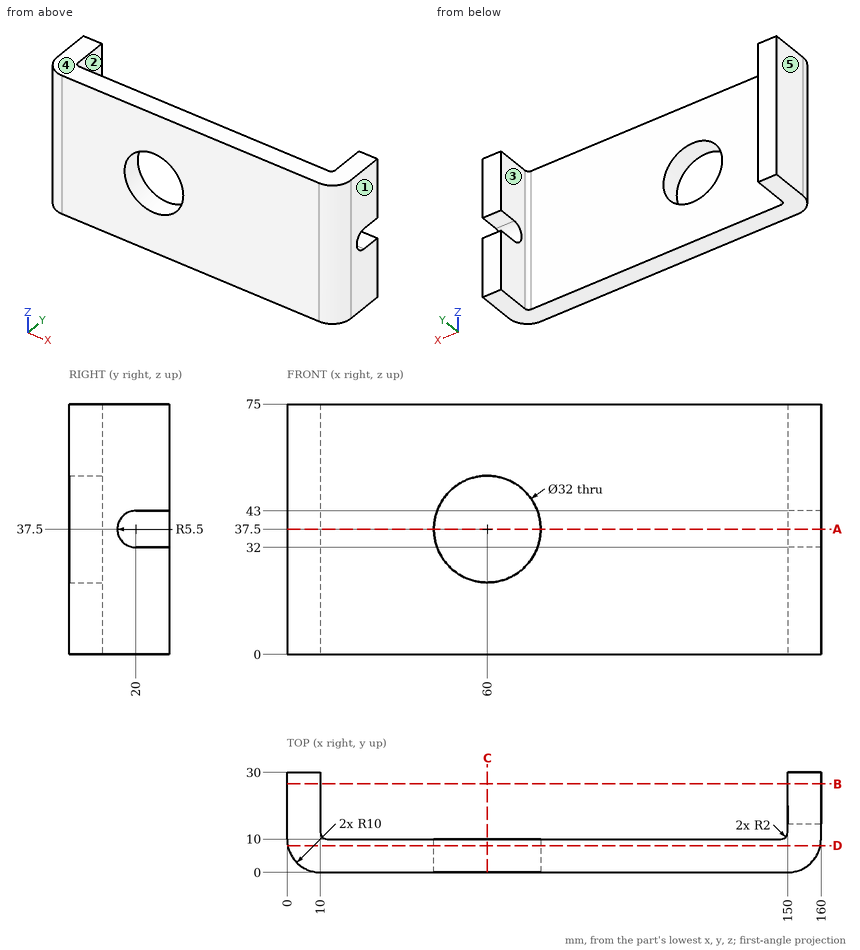
Check sheet for the drawn part. Datum: minimum x, y, z corner. Units: mm. A direction names the side the tool comes from. Give positions to 0.01 mm unless a question says otherwise; leave off trailing zeros. Order: outer loops, then holes, each group sorted by start corner. A loop starts at its lowest first (then second) coordinate and runs counter-clockwise, first axis right, second up. Notation, with made-up numbers: (43.5, 66) -> (85.5, 66) arc R18 ccw to (85.5, 95) -> close; hole circle Ø2 at (32, -14). An arc over 180 degrees is marked (long way). Answer as CSV lines item,"result".
Q1. Access from +Z, -Z, +X, -X, +Y, -Y to the whole of each face (thin tool, end or side, straight path). Record for the marked faces 1 and 2.
Solutions:
face 1,"+Z, -Z, +X, +Y, -Y"
face 2,"+Z, -Z, +Y"
Q2. Release check for a two-part mould opening along X. For the marked faces 3, 4 and 5 record: +X half, -X half, draft (parallel to the pull), parting line (faces both ways), or undercut.
Solutions:
face 3,"undercut"
face 4,"draft"
face 5,"-X half"
Q3. Sectioned sample at B-B on y = 26.5. Record the cut outline in (x, z), plus the area to 3 significant figures.
Solutions:
outline,"(0, 0) -> (10, 0) -> (10, 75) -> (0, 75) -> close; (150, 0) -> (160, 0) -> (160, 32) -> (150, 32) -> close; (150, 43) -> (160, 43) -> (160, 75) -> (150, 75) -> close"
area,"1,390 mm²"
Q4. Scan lines: probe 1 along X at (y, z) = (16.5, 31.5); probe 2 along Z at (x, y) = (60, 7); probe 3 along Y at (x, z) = (40, 49). Record each from-to range of solid material in increasing order.
Solutions:
probe 1,"x = 0 to 10, 150 to 160"
probe 2,"z = 0 to 21.5, 53.5 to 75"
probe 3,"y = 0 to 10"
Q5. Depth check by flat-ended pin: pin 1 (5.5 mm diameter, centred on y = 18.5, z = 38.5, fed in from +X); pin 2 (22.5 mm diameter, centred on x = 77.5, z = 38, fed in from +Y). Enter the tip coordinate at first touch or a pass-through.
Solutions:
pin 1,"stops at x = 10"
pin 2,"stops at y = 10"
Q6. Sectioned sample at D-D on y = 8. Record the cut outline in (x, z).
Solutions:
outline,"(0.2, 0) -> (159.8, 0) -> (159.8, 75) -> (0.2, 75) -> close; hole circle Ø32 at (60, 37.5)"
Q7. Sectioned sample at C-C on x = 60. Record the cut outline in (y, z), plus the area to 3 significant figures.
Solutions:
outline,"(0, 0) -> (10, 0) -> (10, 21.5) -> (0, 21.5) -> close; (0, 53.5) -> (10, 53.5) -> (10, 75) -> (0, 75) -> close"
area,"430 mm²"
Q8. Sectioned sample at A-A on z = 37.5. Record the cut outline in (x, y).
Solutions:
outline,"(0, 10) arc R10 ccw to (10, 0) -> (44, 0) -> (44, 10) -> (12, 10) arc R2 cw to (10, 12) -> (10, 30) -> (0, 30) -> close; (76, 0) -> (150, 0) arc R10 ccw to (160, 10) -> (160, 14.5) -> (150, 14.5) -> (150, 12) arc R2 cw to (148, 10) -> (76, 10) -> close"
